Geometry: final body of the model. Coordinates: model frame, mm. Face numbers are marked on the shaded views. A direction names the side the tool comes from. Give positions to 0.01 mm unless a question says otherwise; leave off trailing zeros. Write each loop counter-clockwise with the first axis right and the second up, starting at its lowest first coordinate (ties: lowest second). Pieces come first, ordered by that corner, then holes.
Q1. Cut plane B-B on x = -39.37. Return the cut outline in (y, z).
Q2. Cut plane D-D on y = -10. Return the cut outline in (x, z), plus the area to 3 significant figures.
Q3. Pin query (flat end, axial travel): pin 1 (2 mm diameter, centred on x = -5.5, z = 15, fed in from +Y); pin 2 (15 mm diameter, centred on x = -2.5, y = -2, fed in from +Z); pin 3 (4 mm diameter, centred on x = 25.65, z = 31.7, fed in from +Y). Return the tip coordinate at first contact, or that it passes through.
Q4. Cut plane A-A on z = 59. Return the cut outline in (x, y).
Q5. Cut plane C-C on x = 27.5. Return the cut outline in (y, z).
Q6. Reachability of the marked faces 1 and 2 from +Z, -Z, +X, -X, +Y, -Y: full face, straight path, thin tool, end or side. Return the list, or none.
Q7. Line query: L1, parallel to Z at x = -39.37, y = -15; L2, parallel to Z at x = -28.5, y = -10; L3, parallel to Y at x = 29, z = 30.5. Output: solid intervals per line, ascending.
```python
from build123d import *

# Parameters (mm, degrees)
F0_W     = 88.9
F0_H     = 31.115
F1_DEPTH = 1.2192
F2_W     = 88.9
F2_H     = 1.2192
F3_DEPTH = 119.38
F4_R     = 0.0508
F5_R     = 3.3401
F6_DEPTH = 25.4


with BuildPart() as f1:
    # F0 (on Top) → F1 (new body)
    with BuildSketch(Plane.XY):
        Rectangle(F0_W, F0_H)
    extrude(amount=F1_DEPTH)

    # F2 (on face) → F3 (join)
    with BuildSketch(Plane.XY.offset(1.2192)):
        with Locations((0, -14.9479)):
            Rectangle(F2_W, F2_H)
    extrude(amount=F3_DEPTH)

    # F4
    f4_edges = [f1.edges().sort_by_distance(p)[0] for p in [
        (0, -15.5575, 0),
        (0, -14.3383, 1.2192),
    ]]
    fillet(f4_edges, radius=F4_R)

    # F5 (on face) → F6 (cut)
    with BuildSketch(Plane.XZ.offset(15.5575)):
        with Locations((21.59, 110.4392)):
            Circle(F5_R)
        with Locations((25.654, 31.6992)):
            Circle(F5_R)
        with Locations((-39.37, 57.0992)):
            Circle(F5_R)
    extrude(amount=-F6_DEPTH, mode=Mode.SUBTRACT)


solid = f1.part
```
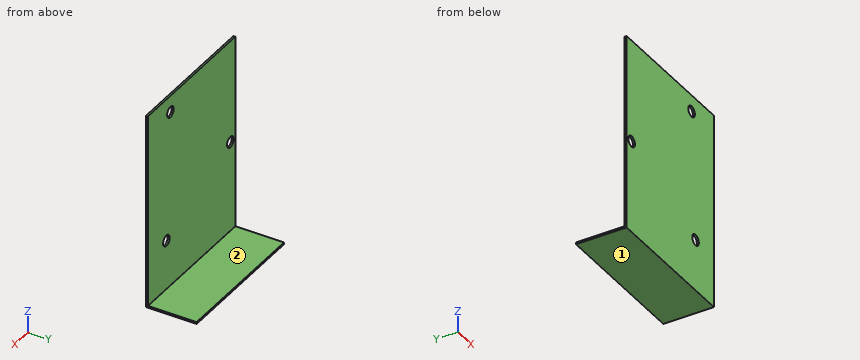
Data:
1. outline: (-15.56, 0.05) arc R0.05 ccw to (-15.51, 0) - (15.56, 0) - (15.56, 1.22) - (-14.29, 1.22) arc R0.05 cw to (-14.34, 1.27) - (-14.34, 53.76) - (-15.56, 53.76) - close; (-15.56, 60.44) - (-14.34, 60.44) - (-14.34, 120.6) - (-15.56, 120.6) - close
2. outline: (-44.45, 0) - (44.45, 0) - (44.45, 1.22) - (-44.45, 1.22) - close
2. area: 108 mm2
3. pin 1: stops at y = -14.34
3. pin 2: stops at z = 1.22
3. pin 3: passes through
4. outline: (-44.45, -15.56) - (-42.12, -15.56) - (-42.12, -14.34) - (-44.45, -14.34) - close; (-36.62, -15.56) - (44.45, -15.56) - (44.45, -14.34) - (-36.62, -14.34) - close
5. outline: (-15.56, 0.05) arc R0.05 ccw to (-15.51, 0) - (15.56, 0) - (15.56, 1.22) - (-14.29, 1.22) arc R0.05 cw to (-14.34, 1.27) - (-14.34, 28.92) - (-15.56, 28.92) - close; (-15.56, 34.48) - (-14.34, 34.48) - (-14.34, 120.6) - (-15.56, 120.6) - close
6. face 1: -Z, +X, -X, +Y, -Y
6. face 2: +Z, +X, -X, +Y
7. L1: z = 0 to 53.76, 60.44 to 120.6
7. L2: z = 0 to 1.22
7. L3: y = -15.56 to -14.34
